```python
from build123d import *

# Parameters (mm, degrees)
PAD_DEPTH       = 80
PAD_DEPTH_BACK  = 20
SKETCH001_R     = 2.6
SKETCH001_R_2   = 1.6
SKETCH001_R_3   = 0.5
POCKET_DEPTH    = 18.001
SKETCH002_W     = 62.404188
SKETCH002_H     = 27.650393
POCKET001_DEPTH = 13
POCKET002_DEPTH = 5
SKETCH004_R     = 10.65
POCKET003_DEPTH = 30.4
SKETCH005_R     = 10.65
POCKET004_DEPTH = 30.4
FILLET_R        = 5
CHAMFER_SIZE    = 2


with BuildPart() as part:
    # Sketch → Pad (new body, two sides)
    with BuildSketch(Plane.XZ) as pad_sk:
        with BuildLine():
            Line((-77.5, -18), (-77.5, -13))
            Line((-77.5, -13), (-22.5, -13))
            Line((-22.5, -13), (-22.5, 0))
            Line((-7, 0), (-22.5, 0))
            ThreePointArc((-7, 0), (0, -7), (7, 0))
            Line((7, 0), (22.5, 0))
            Line((22.5, 0), (22.5, -18))
            Line((22.5, -18), (-77.5, -18))
        make_face()
    extrude(amount=PAD_DEPTH)
    extrude(pad_sk.sketch, amount=-PAD_DEPTH_BACK)

    # Sketch001 → Pocket (cut, through all)
    with BuildSketch(Plane.XY):
        with Locations((-67.5, 10)):
            Circle(SKETCH001_R)
        with Locations((-27.5, 10)):
            Circle(SKETCH001_R)
        with Locations((12.5, 10)):
            Circle(SKETCH001_R)
        with Locations((-17.5, -5)):
            Circle(SKETCH001_R_2)
        with Locations((-17.5, -40)):
            Circle(SKETCH001_R_2)
        with Locations((-17.5, -75)):
            Circle(SKETCH001_R_2)
        with Locations((17.5, -5)):
            Circle(SKETCH001_R_2)
        with Locations((17.5, -40)):
            Circle(SKETCH001_R_2)
        with Locations((17.5, -75)):
            Circle(SKETCH001_R_2)
        with Locations((0, 20)):
            Circle(SKETCH001_R_3)
        Polygon((-77.5, 0), (-77.5, -80), (-22.5, -80), align=None)
    extrude(amount=-POCKET_DEPTH, mode=Mode.SUBTRACT)

    # Sketch002 → Pocket001 (cut)
    with BuildSketch(Plane.XY):
        with Locations((0, 13.825196)):
            Rectangle(SKETCH002_W, SKETCH002_H)
    extrude(amount=-POCKET001_DEPTH, mode=Mode.SUBTRACT)

    # Sketch003 (on DatumPlane) → Pocket002 (cut)
    with BuildSketch(Plane.XY.offset(-18)):
        Polygon((-14.7, -3.383419), (-17.5, -1.766838), (-20.3, -3.383419), (-20.3, -6.616581), (-17.5, -8.233162), (-14.7, -6.616581), align=None)
        Polygon((-14.7, -41.616581), (-14.7, -38.383419), (-17.5, -36.766838), (-20.3, -38.383419), (-20.3, -41.616581), (-17.5, -43.233162), align=None)
        Polygon((-14.7, -76.616581), (-14.7, -73.383419), (-17.5, -71.766838), (-20.3, -73.383419), (-20.3, -76.616581), (-17.5, -78.233162), align=None)
        Polygon((17.5, -78.233162), (20.3, -76.616581), (20.3, -73.383419), (17.5, -71.766838), (14.7, -73.383419), (14.7, -76.616581), align=None)
        Polygon((20.3, -41.616581), (20.3, -38.383419), (17.5, -36.766838), (14.7, -38.383419), (14.7, -41.616581), (17.5, -43.233162), align=None)
        Polygon((20.3, -3.383419), (17.5, -1.766838), (14.7, -3.383419), (14.7, -6.616581), (17.5, -8.233162), (20.3, -6.616581), align=None)
    extrude(amount=POCKET002_DEPTH, mode=Mode.SUBTRACT)

    # Sketch004 (on DatumPlane) → Pocket003 (cut)
    with BuildSketch(Plane.XZ.offset(5)):
        Circle(SKETCH004_R)
    extrude(amount=POCKET003_DEPTH, mode=Mode.SUBTRACT)

    # Sketch005 (on DatumPlane) → Pocket004 (cut)
    with BuildSketch(Plane.XZ.offset(75)):
        Circle(SKETCH005_R)
    extrude(amount=-POCKET004_DEPTH, mode=Mode.SUBTRACT)

    # Fillet
    fillet_edges = [part.edges().sort_by_distance(p)[0] for p in [
        (22.5, 20, -15.5),
        (-77.5, 20, -15.5),
        (-77.5, 0, -15.5),
        (22.5, -80, -9),
    ]]
    fillet(fillet_edges, radius=FILLET_R)

    # Chamfer
    chamfer_edges = [part.edges().sort_by_distance(p)[0] for p in [
        (-22.5, -40, -13),
        (0, 0, -13),
    ]]
    chamfer(chamfer_edges, length=CHAMFER_SIZE)


solid = part.part
```
Design review of the part built by this model. Coordinates are the model's own, in mm. A direction names the side the tool comes from. Coordinates: 2 decimals unless noted, no trailing zeros. Order: outer loops, then holes, each group sorted by start corner. A loop starts at its lowest first (then second) coordinate and runs counter-clockwise, first axis right, second up. Notation, with made-up numbers: M 21,74.5 L 38,74.5 A13 cw 38,83.5 Z; hole C 51.5,-18 d1. An arc over 180 degrees is marked long. Answer as a JSON object with one key per item and string values. Group by question number.
1) Tool access review of faces 1 (the cylindrical face through (13.7, 7.693, -15.465)), 2 (the flat face through (0, -5, -8)), 3 (the flat face through (-16.08, -2.586, -15.535)): name each direction out of +Z, -Z, +X, -X, +Y, -Y from which nothing blocks a thin tool from reaching the whole face with its end or side.
2) Mouldability with a two-part tool opening along X and no side actions: class faces 4 (the flat face through (16.12, -37.564, -15.535)), 5 (the cylindrical face through (21.07, -78.5, -9.13)), 6 (the cylindrical face through (-77.28, 0.09, -15.54)), 7 (the flat face through (9, 20, -15)) as pulls with the +X half, pulls with the -X half, needs draft (parallel to the pull), parting line crosses it, or undercut.
3) Add section C-C, the plane z = -14.25. Count the separate pieces of the cut face and the enclosed holes in it, then the cut area to 3 significant figures.
4) For pin 1 (2.5 mm diameter, centred on y = -5, z = -16, fed in from -X); pin 2 (1.6 mm diameter, centred on y = -5, z = -15, fed in from -X); pin 3 (3.5 mm diameter, centred on y = -41, z = -16.5, fed in from -X), all flat-tipped, find the tip position at first contact; note any pin that passes through.
5) Add section A-A, the plane y = -40. Write out the cut boundary in (x, z), then the cut area to 3 significant figures.
6) Add section B-B, the plane y = -52. Write out the cut boundary in (x, z), then the cut area to 3 significant figures.
7) Wall thickness on L1, parallel to Y at x = -17.5, z = -4.25; L2, parallel to X at y = -9, z = -0.75; L3, parallel to X at y = -74.5, z = -2.5: over which ranges is each line inside the solid? List them lowest first.
8) Add section D-D, the plane x = 5. Write out the cut boundary in (y, z).
Computed values:
{
 "1": {"face 1": "+Z, -Z", "face 2": "+Z", "face 3": "-Z"},
 "2": {"face 4": "undercut", "face 5": "pulls with the +X half", "face 6": "pulls with the -X half", "face 7": "needs draft"},
 "3": {"separate pieces": "1", "enclosed holes": "9", "area": "7,560 mm^2"},
 "4": {"pin 1": "stops at x = -74.92", "pin 2": "stops at x = -74.61", "pin 3": "stops at x = -50.52"},
 "5": {"outline": "M -50,-18 L -20.3,-18 L -20.3,-13 L -19.1,-13 L -19.1,0 L -22.5,0 L -22.5,-11 L -24.5,-13 L -50,-13 Z; M -15.9,-13 L -14.7,-13 L -14.7,-18 L 14.7,-18 L 14.7,-13 L 15.9,-13 L 15.9,0 L 7,0 A7 cw -7,0 L -15.9,0 Z; M 19.1,-13 L 20.3,-13 L 20.3,-18 L 22.5,-18 L 22.5,0 L 19.1,0 Z", "area": "733 mm^2"},
 "6": {"outline": "M -41.75,-18 L 22.5,-18 L 22.5,0 L 10.65,0 A10.65 cw -10.65,0 L -22.5,0 L -22.5,-11 L -24.5,-13 L -41.75,-13 Z", "area": "730 mm^2"},
 "7": {"L1": "y = -80 to -76.6, -73.4 to -41.6, -38.4 to -6.6, -3.4 to 0", "L2": "x = -22.5 to -10.62, 10.62 to 22.5", "L3": "x = -22.5 to -19.02, -15.98 to -10.35, 10.35 to 15.98, 19.02 to 22.5"},
 "8": {"outline": "M -80,-18 L 20,-18 L 20,-13 L 2,-13 L 0,-11 L 0,-4.9 L -5,-4.9 L -5,-9.4 L -35.4,-9.4 L -35.4,-4.9 L -44.6,-4.9 L -44.6,-9.4 L -75,-9.4 L -75,-4.9 L -80,-4.9 Z"}
}
